from build123d import *

# Parameters (mm, degrees)
SKETCH3_W                  = 100
SKETCH3_H                  = 100
BOSS_EXTRUDE2_DEPTH        = 4
SKETCH4_W                  = 8.5
SKETCH4_H                  = 8.5
CUT_EXTRUDE1_DEPTH         = 142.477913471
CUT_EXTRUDE2_DEPTH         = 142.477913471
FILLET4_R                  = 4
FILLET6_R                  = 4
BOSS_EXTRUDE3_DEPTH        = 3
M2X0_4_TAPPED_HOLE1_D      = 1.6
M2X0_4_TAPPED_HOLE1_DEPTH  = 5.2
M2X0_4_TAPPED_HOLE1_TIP    = 0.480688495
M2X0_4_TAPPED_HOLE2_REACH  = 143.478
M2X0_4_TAPPED_HOLE2_BORE_R = 0.8
M2X0_4_TAPPED_HOLE3_D      = 1.6
M2X0_4_TAPPED_HOLE3_DEPTH  = 8.52
M2X0_4_TAPPED_HOLE3_TIP    = 0.480688495
M2X0_4_TAPPED_HOLE13_D     = 1.6
M2X0_4_TAPPED_HOLE5_D      = 1.6
M2X0_4_TAPPED_HOLE5_DEPTH  = 6
M2X0_4_TAPPED_HOLE5_TIP    = 0.480688495
FILLET7_R                  = 4
FILLET8_R                  = 4
M2X0_4_TAPPED_HOLE9_D      = 1.6
M2X0_4_TAPPED_HOLE9_DEPTH  = 6
M2X0_4_TAPPED_HOLE9_TIP    = 0.480688495
M2X0_4_TAPPED_HOLE10_D     = 1.6
M2X0_4_TAPPED_HOLE10_DEPTH = 6
M2X0_4_TAPPED_HOLE10_TIP   = 0.480688495
SKETCH33_W                 = 83
SKETCH33_H                 = 1.6
SKETCH33_W_2               = 1.6
SKETCH33_H_2               = 83
CUT_EXTRUDE3_DEPTH         = 10
M2X0_4_TAPPED_HOLE11_D     = 1.6
M2X0_4_TAPPED_HOLE11_DEPTH = 6
M2X0_4_TAPPED_HOLE11_TIP   = 0.480688495
M2X0_4_TAPPED_HOLE12_D     = 1.6
M2X0_4_TAPPED_HOLE12_DEPTH = 6
M2X0_4_TAPPED_HOLE12_TIP   = 0.480688495


with BuildPart() as part:
    # Sketch3 → Boss-Extrude2 (new body)
    with BuildSketch(Plane.XY):
        with Locations((50, -50)):
            Rectangle(SKETCH3_W, SKETCH3_H)
    extrude(amount=BOSS_EXTRUDE2_DEPTH)

    # Sketch4 → Cut-Extrude1 (cut, through all)
    with BuildSketch(Plane(origin=(0, 0, 0), x_dir=(-1, 0, 0), z_dir=(0, 0, -1))):
        with Locations((-4.25, -95.75)):
            Rectangle(SKETCH4_W, SKETCH4_H)
        with Locations((-4.25, -4.25)):
            Rectangle(SKETCH4_W, SKETCH4_H)
        with Locations((-95.75, -4.25)):
            Rectangle(SKETCH4_W, SKETCH4_H)
        with Locations((-95.75, -95.75)):
            Rectangle(SKETCH4_W, SKETCH4_H)
    extrude(amount=-CUT_EXTRUDE1_DEPTH, mode=Mode.SUBTRACT)

    # Sketch5 → Cut-Extrude2 (cut, through all)
    with BuildSketch(Plane(origin=(0, 0, 0), x_dir=(-1, 0, 0), z_dir=(0, 0, -1))):
        Polygon((-94, -14.5), (-85.5, -14.5), (-85.5, -6), (-14.5, -6), (-14.5, -14.5), (-6, -14.5), (-6, -85.5), (-14.5, -85.5), (-14.5, -94), (-85.5, -94), (-85.5, -85.5), (-94, -85.5), align=None)
    extrude(amount=-CUT_EXTRUDE2_DEPTH, mode=Mode.SUBTRACT)

    # Fillet4
    fillet4_edges = [part.edges().sort_by_distance(p)[0] for p in [
        (85.5, -14.5, 2),
        (14.5, -14.5, 2),
        (14.5, -85.5, 2),
        (85.5, -85.5, 2),
    ]]
    fillet(fillet4_edges, radius=FILLET4_R)

    # Fillet6
    fillet6_edges = [part.edges().sort_by_distance(p)[0] for p in [
        (94, -85.5, 2),
        (94, -14.5, 2),
        (85.5, -6, 2),
        (14.5, -6, 2),
        (6, -14.5, 2),
        (6, -85.5, 2),
        (14.5, -94, 2),
        (85.5, -94, 2),
    ]]
    fillet(fillet6_edges, radius=FILLET6_R)

    # Sketch6 → Boss-Extrude3 (add)
    with BuildSketch(Plane.XY.offset(4)):
        with BuildLine():
            Line((6, -45), (6, -55))
            ThreePointArc((6, -55), (11, -50), (6, -45))
        make_face()
        with BuildLine():
            Line((94, -45), (94, -55))
            ThreePointArc((94, -55), (89, -50), (94, -45))
        make_face()
        with BuildLine():
            Line((45, -6), (55, -6))
            ThreePointArc((55, -6), (50, -11), (45, -6))
        make_face()
        with BuildLine():
            Line((45, -94), (55, -94))
            ThreePointArc((55, -94), (50, -89), (45, -94))
        make_face()
    extrude(amount=-BOSS_EXTRUDE3_DEPTH)

    # M2x0.4 Tapped Hole1
    with Locations(Plane.XY.offset(4)):
        with Locations((50, -3.8), (3.8, -12.5), (50, -96.2), (96.2, -87.5), (3.8, -87.5), (96.2, -12.5)):
            Hole(M2X0_4_TAPPED_HOLE1_D / 2, depth=M2X0_4_TAPPED_HOLE1_DEPTH)
            with Locations((0, 0, -(M2X0_4_TAPPED_HOLE1_DEPTH + M2X0_4_TAPPED_HOLE1_TIP / 2))):  # 118° drill point
                Cone(0, M2X0_4_TAPPED_HOLE1_D / 2, M2X0_4_TAPPED_HOLE1_TIP, mode=Mode.SUBTRACT)

    # M2x0.4 Tapped Hole2 bore → M2x0.4 Tapped Hole2 (cut, up to next)
    with BuildSketch(Plane(origin=(0, 0, 0), x_dir=(1, 0, 0), z_dir=(0, 1, 0)), mode=Mode.PRIVATE) as m2x0_4_tapped_hole2_sk1:
        with Locations((83.5, -2)):
            Circle(M2X0_4_TAPPED_HOLE2_BORE_R)
    m2x0_4_tapped_hole2_tool1 = extrude(m2x0_4_tapped_hole2_sk1.sketch, amount=-M2X0_4_TAPPED_HOLE2_REACH, mode=Mode.PRIVATE) & part.part
    # M2x0.4 Tapped Hole2 bore → M2x0.4 Tapped Hole2 (cut, up to next)
    with BuildSketch(Plane(origin=(0, 0, 0), x_dir=(1, 0, 0), z_dir=(0, 1, 0)), mode=Mode.PRIVATE) as m2x0_4_tapped_hole2_sk2:
        with Locations((16.5, -2)):
            Circle(M2X0_4_TAPPED_HOLE2_BORE_R)
    m2x0_4_tapped_hole2_tool2 = extrude(m2x0_4_tapped_hole2_sk2.sketch, amount=-M2X0_4_TAPPED_HOLE2_REACH, mode=Mode.PRIVATE) & part.part
    add(m2x0_4_tapped_hole2_tool1.solids().sort_by_distance((83.5, 0, 2))[0], mode=Mode.SUBTRACT)
    add(m2x0_4_tapped_hole2_tool2.solids().sort_by_distance((16.5, 0, 2))[0], mode=Mode.SUBTRACT)

    # M2x0.4 Tapped Hole3
    with Locations(Plane(origin=(100, 0, 0), x_dir=(0, 0, -1), z_dir=(1, 0, 0))):
        with Locations((-2, -83.5), (-2, -16.5)):
            Hole(M2X0_4_TAPPED_HOLE3_D / 2, depth=M2X0_4_TAPPED_HOLE3_DEPTH)
            with Locations((0, 0, -(M2X0_4_TAPPED_HOLE3_DEPTH + M2X0_4_TAPPED_HOLE3_TIP / 2))):  # 118° drill point
                Cone(0, M2X0_4_TAPPED_HOLE3_D / 2, M2X0_4_TAPPED_HOLE3_TIP, mode=Mode.SUBTRACT)

    # M2x0.4 Tapped Hole13 (through all)
    with Locations(Plane.ZY):
        with Locations((2, -83.5), (2, -16.5)):
            Hole(M2X0_4_TAPPED_HOLE13_D / 2)

    # M2x0.4 Tapped Hole5
    with Locations(Plane(origin=(0, -100, 0), x_dir=(-1, 0, 0), z_dir=(0, -1, 0))):
        with Locations((-16.5, -2), (-83.5, -2)):
            Hole(M2X0_4_TAPPED_HOLE5_D / 2, depth=M2X0_4_TAPPED_HOLE5_DEPTH)
            with Locations((0, 0, -(M2X0_4_TAPPED_HOLE5_DEPTH + M2X0_4_TAPPED_HOLE5_TIP / 2))):  # 118° drill point
                Cone(0, M2X0_4_TAPPED_HOLE5_D / 2, M2X0_4_TAPPED_HOLE5_TIP, mode=Mode.SUBTRACT)

    # Fillet7
    fillet7_edges = [part.edges().sort_by_distance(p)[0] for p in [
        (6, -45, 2.5),
    ]]
    fillet(fillet7_edges, radius=FILLET7_R)

    # Fillet8
    fillet8_edges = [part.edges().sort_by_distance(p)[0] for p in [
        (6, -55, 2.5),
        (94, -55, 2.5),
        (94, -45, 2.5),
        (55, -6, 2.5),
        (45, -6, 2.5),
        (45, -94, 2.5),
        (55, -94, 2.5),
    ]]
    fillet(fillet8_edges, radius=FILLET8_R)

    # M2x0.4 Tapped Hole9
    with Locations(Plane.ZY.offset(-8.5)):
        with Locations((2, -95.75)):
            Hole(M2X0_4_TAPPED_HOLE9_D / 2, depth=M2X0_4_TAPPED_HOLE9_DEPTH)
            with Locations((0, 0, -(M2X0_4_TAPPED_HOLE9_DEPTH + M2X0_4_TAPPED_HOLE9_TIP / 2))):  # 118° drill point
                Cone(0, M2X0_4_TAPPED_HOLE9_D / 2, M2X0_4_TAPPED_HOLE9_TIP, mode=Mode.SUBTRACT)

    # M2x0.4 Tapped Hole10
    with Locations(Plane.ZY.offset(-8.5)):
        with Locations((2, -4.25)):
            Hole(M2X0_4_TAPPED_HOLE10_D / 2, depth=M2X0_4_TAPPED_HOLE10_DEPTH)
            with Locations((0, 0, -(M2X0_4_TAPPED_HOLE10_DEPTH + M2X0_4_TAPPED_HOLE10_TIP / 2))):  # 118° drill point
                Cone(0, M2X0_4_TAPPED_HOLE10_D / 2, M2X0_4_TAPPED_HOLE10_TIP, mode=Mode.SUBTRACT)

    # Sketch33 → Cut-Extrude3 (cut)
    with BuildSketch(Plane.XY.offset(4)):
        with Locations((50, -99.2)):
            Rectangle(SKETCH33_W, SKETCH33_H)
        with Locations((99.2, -50)):
            Rectangle(SKETCH33_W_2, SKETCH33_H_2)
        with Locations((50, -0.8)):
            Rectangle(SKETCH33_W, SKETCH33_H)
        with Locations((0.8, -50)):
            Rectangle(SKETCH33_W_2, SKETCH33_H_2)
    extrude(amount=-CUT_EXTRUDE3_DEPTH, mode=Mode.SUBTRACT)

    # M2x0.4 Tapped Hole11
    with Locations(Plane(origin=(91.5, 0, 0), x_dir=(0, 0, -1), z_dir=(1, 0, 0))):
        with Locations((-2, -95.75)):
            Hole(M2X0_4_TAPPED_HOLE11_D / 2, depth=M2X0_4_TAPPED_HOLE11_DEPTH)
            with Locations((0, 0, -(M2X0_4_TAPPED_HOLE11_DEPTH + M2X0_4_TAPPED_HOLE11_TIP / 2))):  # 118° drill point
                Cone(0, M2X0_4_TAPPED_HOLE11_D / 2, M2X0_4_TAPPED_HOLE11_TIP, mode=Mode.SUBTRACT)

    # M2x0.4 Tapped Hole12
    with Locations(Plane(origin=(91.5, 0, 0), x_dir=(0, 0, -1), z_dir=(1, 0, 0))):
        with Locations((-2, -4.25)):
            Hole(M2X0_4_TAPPED_HOLE12_D / 2, depth=M2X0_4_TAPPED_HOLE12_DEPTH)
            with Locations((0, 0, -(M2X0_4_TAPPED_HOLE12_DEPTH + M2X0_4_TAPPED_HOLE12_TIP / 2))):  # 118° drill point
                Cone(0, M2X0_4_TAPPED_HOLE12_D / 2, M2X0_4_TAPPED_HOLE12_TIP, mode=Mode.SUBTRACT)


solid = part.part
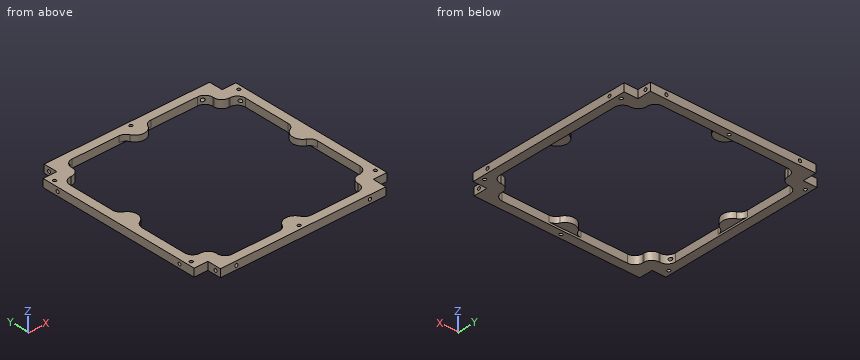
CAD build for the part. Positions are in the model's coordinates, mm. Round coordinates to 2 decimals unless told otherwise and drop trailing zeros. Write each loop counter-clockwise with the first axis right and the second up, starting at its lowest first coordinate (ties: lowest second). Pieces come first, ordered by that corner, then holes.
(1) Slice it at A-A, the plane x = 79. Write the cut outline in (y, z).
(2) Drop flat-ended pins along their axis: P1, Ø1.5, axis at x = 51.5, y = -92, coming from the -Z side; P2, Ø1, axis at y = -95.75, z = 2, coming from the -X side; P3, Ø2, axis at x = 50, y = -3.8, coming from the -Z side; P4, Ø1.4, axis at y = -4.25, z = 2, coming from the +X side. Give the stop position or say it passes through.
(3) Probe line 1 along Z through (x, y) = (87.05, -95.75); line 2 along X through (y, z) = (-25, 2.1); line 3 along Y through (x, z) = (95.3, 2). List the from-to ranges inside material, lowest first.
(4) Slice it at B-B, the plane y = -50. Write the cut outline in (x, z).
(5) Slice it at D-D, the plane y = -36. Write the cut outline in (x, z), and give its area (3 significant figures).
(6) Slice it at C-C, the plane x = 12.5. Write the cut outline in (y, z).
From the geometry:
1. outline: (-98.4, 0) - (-94, 0) - (-94, 4) - (-98.4, 4) - close; (-6, 0) - (-1.6, 0) - (-1.6, 4) - (-6, 4) - close
2. P1: stops at z = 1
2. P2: stops at x = 14.68
2. P3: stops at z = 0
2. P4: stops at x = 85.44
3. line 1: z = 0 to 1.2, 2.8 to 4
3. line 2: x = 1.6 to 6, 94 to 98.4
3. line 3: y = -91.5 to -84.3, -82.7 to -17.3, -15.7 to -8.5
4. outline: (1.6, 0) - (6, 0) - (6, 1) - (11, 1) - (11, 4) - (1.6, 4) - close; (89, 1) - (94, 1) - (94, 0) - (98.4, 0) - (98.4, 4) - (89, 4) - close
5. outline: (1.6, 0) - (6, 0) - (6, 4) - (1.6, 4) - close; (94, 0) - (98.4, 0) - (98.4, 4) - (94, 4) - close
5. area: 35.2 mm2
6. outline: (-98.4, 0) - (-86.04, 0) - (-86.04, 4) - (-98.4, 4) - close; (-13.96, 0) - (-1.6, 0) - (-1.6, 4) - (-13.96, 4) - close; hole circle Ø1.6 at (-95.75, 2); hole circle Ø1.6 at (-4.25, 2)
